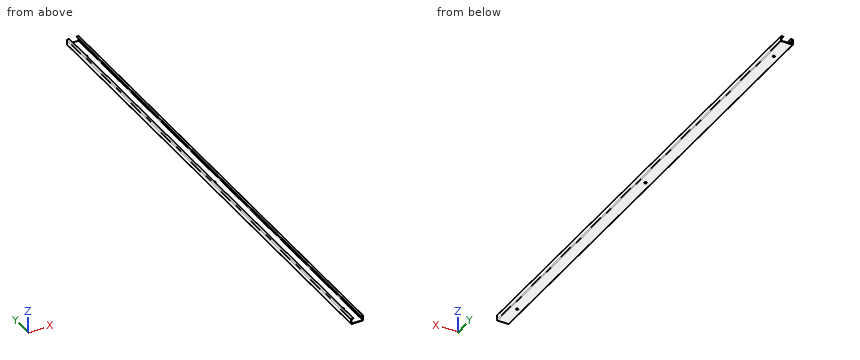
```python
from build123d import *

# Parameters (mm, degrees)
BASEFLANGE_W                   = 50
BASEFLANGE_H                   = 2047
BASE_FLANGE1_DEPTH             = 2
EDGE_FLANGE1_STRIP_W           = 10
EDGE_FLANGE1_STRIP_H           = 2
EDGE_FLANGE1_STRIP_CUT_DEPTH   = 2047
EDGE_FLANGE1_STRIP_2_W         = 10
EDGE_FLANGE1_STRIP_2_H         = 2
EDGE_FLANGE1_STRIP_CUT_2_DEPTH = 2047
EDGE_FLANGE1_DEPTH             = 2047
EDGE_FLANGE1_BEND_DEPTH        = 2047
EDGE_FLANGE2_STRIP_W           = 10
EDGE_FLANGE2_STRIP_H           = 2
EDGE_FLANGE2_STRIP_CUT_DEPTH   = 2047
EDGE_FLANGE2_STRIP_2_W         = 10
EDGE_FLANGE2_STRIP_2_H         = 2
EDGE_FLANGE2_STRIP_CUT_2_DEPTH = 2047
EDGE_FLANGE2_DEPTH             = 2047
EDGE_FLANGE2_BEND_DEPTH        = 2047
HINGEHOLES_R                   = 4.6
CUT_EXTRUDE1_DEPTH             = 1025.041625131


# Sheet-metal steps are written as plain solids
with BuildPart() as part:
    # BaseFlange → Base-Flange1 (new body)
    with BuildSketch(Plane.XY):
        Rectangle(BASEFLANGE_W, BASEFLANGE_H)
    extrude(amount=BASE_FLANGE1_DEPTH)

    # Edge-Flange1 strip (across the edge) → Edge-Flange1 strip cut (cut)
    with BuildSketch(Plane(origin=(25, -1023.5, 2), x_dir=(-1, 0, 0), z_dir=(0, 1, 0))):
        with Locations((-2, -1)):
            Rectangle(EDGE_FLANGE1_STRIP_W, EDGE_FLANGE1_STRIP_H)
    extrude(amount=EDGE_FLANGE1_STRIP_CUT_DEPTH, mode=Mode.SUBTRACT)

    # Edge-Flange1 strip 2 (across the edge) → Edge-Flange1 strip cut 2 (cut)
    with BuildSketch(Plane(origin=(-25, 1023.5, 2), x_dir=(1, 0, 0), z_dir=(0, -1, 0))):
        with Locations((-2, -1)):
            Rectangle(EDGE_FLANGE1_STRIP_2_W, EDGE_FLANGE1_STRIP_2_H)
    extrude(amount=EDGE_FLANGE1_STRIP_CUT_2_DEPTH, mode=Mode.SUBTRACT)

    # Edge-Flange1 section (across the edge) → Edge-Flange1 (add)
    with BuildSketch(Plane(origin=(25, -1023.5, 2), x_dir=(-1, 0, 0), z_dir=(0, 1, 0))):
        with BuildLine():
            Line((0, 1), (0, 20))
            Line((0, 20), (2, 20))
            Line((2, 20), (2, 1))
            ThreePointArc((2, 1), (2.292893219, 0.292893219), (3, 0))
            Line((3, 0), (3, -2))
            ThreePointArc((3, -2), (0.878679656, -1.121320344), (0, 1))
        make_face()
    extrude(amount=EDGE_FLANGE1_DEPTH)

    # Edge-Flange1 section 2 (across the edge) → Edge-Flange1 bend (add)
    with BuildSketch(Plane(origin=(-25, 1023.5, 2), x_dir=(1, 0, 0), z_dir=(0, -1, 0))):
        with BuildLine():
            Line((0, 1), (0, 20))
            Line((0, 20), (2, 20))
            Line((2, 20), (2, 1))
            ThreePointArc((2, 1), (2.292893219, 0.292893219), (3, 0))
            Line((3, 0), (3, -2))
            ThreePointArc((3, -2), (0.878679656, -1.121320344), (0, 1))
        make_face()
    extrude(amount=EDGE_FLANGE1_BEND_DEPTH)

    # Edge-Flange2 strip (across the edge) → Edge-Flange2 strip cut (cut)
    with BuildSketch(Plane(origin=(-23, 1023.5, 22), x_dir=(0, 0, -1), z_dir=(0, -1, 0))):
        with Locations((-2, -1)):
            Rectangle(EDGE_FLANGE2_STRIP_W, EDGE_FLANGE2_STRIP_H)
    extrude(amount=EDGE_FLANGE2_STRIP_CUT_DEPTH, mode=Mode.SUBTRACT)

    # Edge-Flange2 strip 2 (across the edge) → Edge-Flange2 strip cut 2 (cut)
    with BuildSketch(Plane(origin=(23, -1023.5, 22), x_dir=(0, 0, -1), z_dir=(0, 1, 0))):
        with Locations((-2, -1)):
            Rectangle(EDGE_FLANGE2_STRIP_2_W, EDGE_FLANGE2_STRIP_2_H)
    extrude(amount=EDGE_FLANGE2_STRIP_CUT_2_DEPTH, mode=Mode.SUBTRACT)

    # Edge-Flange2 section (across the edge) → Edge-Flange2 (add)
    with BuildSketch(Plane(origin=(-23, 1023.5, 22), x_dir=(0, 0, -1), z_dir=(0, -1, 0))):
        with BuildLine():
            Line((0, 1), (0, 8))
            Line((0, 8), (2, 8))
            Line((2, 8), (2, 1))
            ThreePointArc((2, 1), (2.292893219, 0.292893219), (3, 0))
            Line((3, 0), (3, -2))
            ThreePointArc((3, -2), (0.878679656, -1.121320344), (0, 1))
        make_face()
    extrude(amount=EDGE_FLANGE2_DEPTH)

    # Edge-Flange2 section 2 (across the edge) → Edge-Flange2 bend (add)
    with BuildSketch(Plane(origin=(23, -1023.5, 22), x_dir=(0, 0, -1), z_dir=(0, 1, 0))):
        with BuildLine():
            Line((0, 1), (0, 8))
            Line((0, 8), (2, 8))
            Line((2, 8), (2, 1))
            ThreePointArc((2, 1), (2.292893219, 0.292893219), (3, 0))
            Line((3, 0), (3, -2))
            ThreePointArc((3, -2), (0.878679656, -1.121320344), (0, 1))
        make_face()
    extrude(amount=EDGE_FLANGE2_BEND_DEPTH)

    # HingeHoles → Cut-Extrude1 (cut, through all)
    with BuildSketch(Plane.XY):
        with Locations(Location((-2, 925.5, 0), (0, 0, 180))):
            Circle(HINGEHOLES_R)
        with Locations(Location((-2, 0, 0), (0, 0, 180))):
            Circle(HINGEHOLES_R)
        with Locations(Location((-2, -925.5, 0), (0, 0, 180))):
            Circle(HINGEHOLES_R)
    extrude(amount=CUT_EXTRUDE1_DEPTH, mode=Mode.SUBTRACT)


solid = part.part
```
CAD build for the part. Positions are in the model's coordinates, mm. Give positions to 0.01 mm unless a question says otherwise; leave off trailing zeros. Order: outer loops, then holes, each group sorted by start corner. A loop starts at its lowest first (then second) coordinate and runs counter-clockwise, first axis right, second up.
(1) Drill centre lines: L1, parallel to Y at x = -2, z = 1.35; L2, parallel to X at y = -191.5, z = 9.75; L3, parallel to Z at x = 22, y = -26.5. Where is each one in solid material? Low to high.
(2) Saw through at A-A, the plane z = 11.5. Give the cut face in (x, y).
(3) Flat gauge pins, fed straight in: pin 1 (14.5 mm diameter, centred on x = -2, y = 925.5, fed in from +Z); pin 2 (2 mm diameter, centred on y = -198, z = 21, fed in from +X); pin 3 (1 mm diameter, centred on y = -457, z = 21, fed in from -X). Where does each tip first touch, or does it go through?
(4) Saw through at B-B, the plane y = -466.5. Give the cut face in (x, z), then the cut area to 3 significant figures.
Results found:
1. L1: y = -1023.5 to -930.1, -920.9 to -4.6, 4.6 to 920.9, 930.1 to 1023.5
1. L2: x = -25 to -23, 23 to 25
1. L3: z = 0 to 2, 20 to 22
2. outline: (-25, -1023.5) - (-23, -1023.5) - (-23, 1023.5) - (-25, 1023.5) - close; (23, -1023.5) - (25, -1023.5) - (25, 1023.5) - (23, 1023.5) - close
3. pin 1: stops at z = 2
3. pin 2: stops at x = 24.83
3. pin 3: stops at x = -24.6
4. outline: (-25, 3) arc R3 ccw to (-22, 0) - (22, 0) arc R3 ccw to (25, 3) - (25, 19) arc R3 ccw to (22, 22) - (15, 22) - (15, 20) - (22, 20) arc R1 cw to (23, 19) - (23, 3) arc R1 cw to (22, 2) - (-22, 2) arc R1 cw to (-23, 3) - (-23, 19) arc R1 cw to (-22, 20) - (-15, 20) - (-15, 22) - (-22, 22) arc R3 ccw to (-25, 19) - close
4. area: 205 mm2
